Drawing for the job (mm, zero at the part's lowest x, y, z). Round coordinates to 2 decimals unless told otherwise and drop trailing zeros. Order: outer loops, then holes, each group sorted by start corner. A loop starts at its lowest first (then second) coordinate and runs counter-clockwise, first axis right, second up. Notation, with made-up numbers: (63, 43.25) - (106, 43.25) arc R26 ccw to (106, 60.25) - close; hole circle Ø7 at (83, -7). An arc over 180 degrees is marked (long way). One line per question, with ' | ' between items. Start each with the question number.
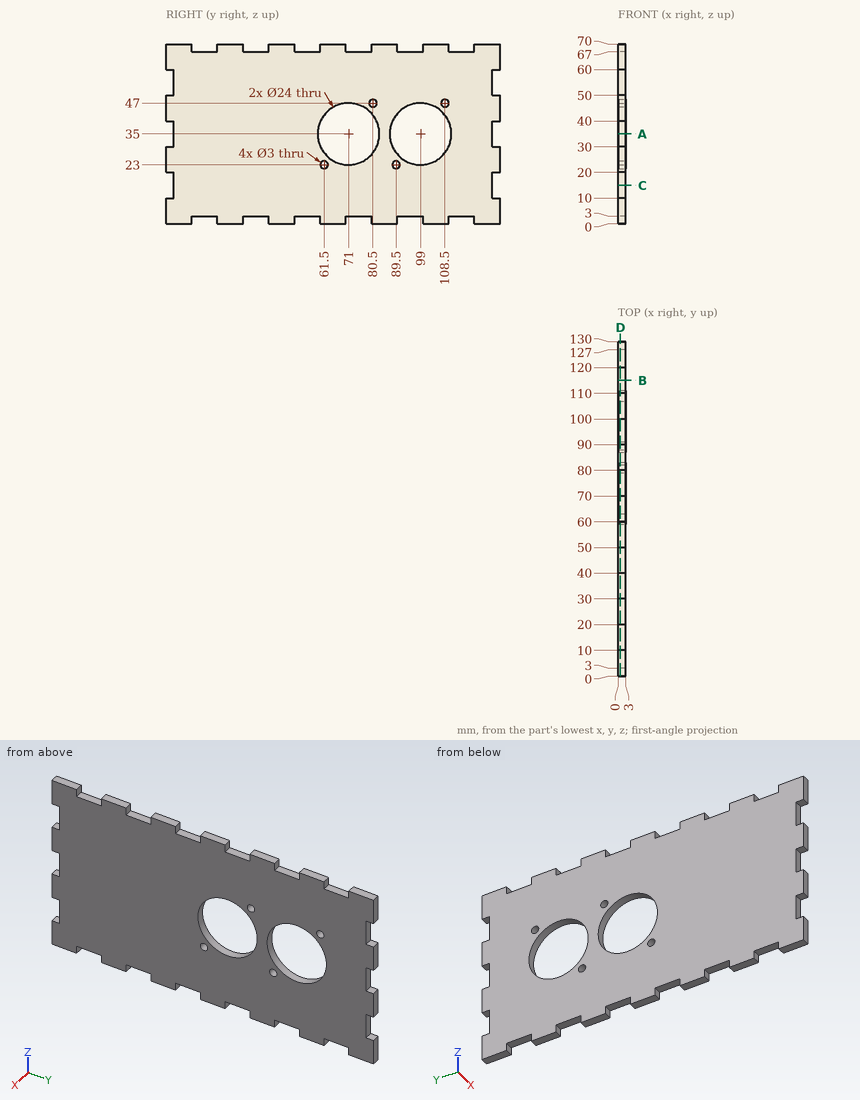
Item 1: Wall check: line 1 along Z through (x, y) = (0.8, 99); line 2 along Z through (x, y) = (0.6, 89.5); line 3 along Y through (x, z) = (2.25, 32.5). Give the ranges that are in metal, low to high. Write a range as [from, to].
Item 2: Slice it at C-C (z = 15). Write the cut outline in (x, y), plus the area to 3 significant figures.
Item 3: Slice it at D-D (x = 0.8). Count the separate pieces of the cut face and the enclosed holes in it, plus the area to 3 significant figures.
Item 4: Slice it at A-A (z = 35). Write the cut outline in (x, y).
Item 5: Slice it at B-B (y = 115). Write the cut outline in (x, z), plus the area to 3 significant figures.
Item 6: Pin check, flat tips, straight feed: pin 1 (1.5 mm diameter, centred on x = 2, z = 17.5, fed in from -Y); pin 2 (14.5 mm diameter, centred on y = 99, z = 35, fed in from -X); pin 3 (0.9 mm diameter, centred on x = 1, y = 53.5, fed in from +Z); pin 4 (0.9 mm diameter, centred on x = 1.5, y = 16, fed in from -Z). Stop position of each tip, or through.
A:
1) line 1: [3, 23], [47, 67] | line 2: [0, 21.5], [24.5, 27.67], [42.33, 70] | line 3: [3, 59.26], [82.74, 87.26], [110.74, 127]
2) outline: (0, 3) - (3, 3) - (3, 127) - (0, 127) - close | area: 372 mm^2
3) separate pieces: 1 | enclosed holes: 6 | area: 7,630 mm^2
4) outline: (0, 3) - (3, 3) - (3, 59) - (0, 59) - close; (0, 83) - (3, 83) - (3, 87) - (0, 87) - close; (0, 111) - (3, 111) - (3, 127) - (0, 127) - close
5) outline: (0, 3) - (3, 3) - (3, 67) - (0, 67) - close | area: 192 mm^2
6) pin 1: y = 3 | pin 2: through | pin 3: z = 67 | pin 4: z = 3
